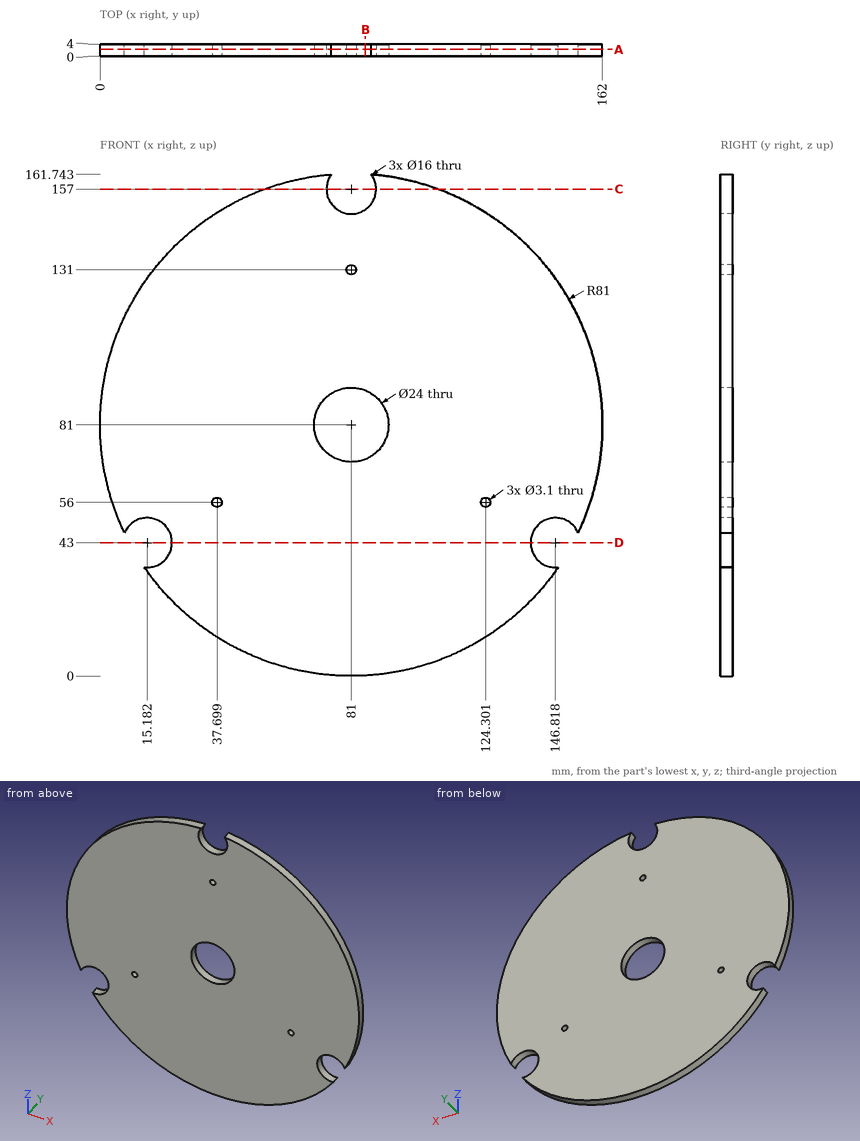
For this review, use the dimensioned drawing (mm, ordinates from the lowest corner) and the shaded views. Give positions to 0.01 mm unless a question says otherwise; leave off trailing zeros. Order: outer loops, then holes, each group sorted by start corner. A loop starts at its lowest first (then second) coordinate and runs counter-clockwise, first axis right, second up.
1) Take a section at C-C (z = 157). Give the boundary of the cut face in (x, y).
2) Take a section at B-B (x = 85.5). Give the boundary of the cut face in (y, z) (1 decimal).
3) Take a section at D-D (z = 43). Give the boundary of the cut face in (x, y).
4) Wall thickness on line 1 (X direction, y = 2.05, z = 81); line 2 (X direction, y = 3.05, z = 43); line 3 (Z direction, x = 124.5, y = 0.65): over which ranges is each line inside the solid? List them lowest first.
5) Take a section at A-A (y = 2.25). State how many separate pieces and enclosed holes the cut face has, then the cut area to 3 significant figures.
6) Insertion check: pin 1 (3.5 mm diameter, centred on x = 81, z = 131, fed in from +Y); pin 2 (1 mm diameter, centred on x = 50, y = 1, fed in from +Z); pin 3 (2 mm diameter, centred on x = 28.5, y = 1.5, fed in from +Z); pin 4 (2 mm diameter, centred on x = 98, y = 3, fed in from -Z). Each pin has a flat end and moves straight along its axis. Give the tip position at first contact, or say it passes through.
Derived:
1. outline: (52.98, 0) - (73, 0) - (73, 4) - (52.98, 4) - close; (89, 0) - (109.02, 0) - (109.02, 4) - (89, 4) - close
2. outline: (0, 0.1) - (4, 0.1) - (4, 69.9) - (0, 69.9) - close; (0, 92.1) - (4, 92.1) - (4, 150.4) - (0, 150.4) - close
3. outline: (23.18, 0) - (138.82, 0) - (138.82, 4) - (23.18, 4) - close
4. line 1: x = 0 to 69, 93 to 162
4. line 2: x = 23.18 to 138.82
4. line 3: z = 12.67 to 54.46, 57.54 to 149.33
5. separate pieces: 1
5. enclosed holes: 4
5. area: 19,600 mm2
6. pin 1: stops at y = 4
6. pin 2: stops at z = 156.04
6. pin 3: stops at z = 143.52
6. pin 4: stops at z = 1.6
